from build123d import *

# Parameters (mm, degrees)
BOSS_EXTRUDE1_DEPTH     = 10
SKETCH4_W               = 12
SKETCH4_H               = 57
BOSS_EXTRUDE2_DEPTH     = 10
SKETCH3_R               = 1.3
CUT_EXTRUDE1_DEPTH      = 1
CUT_EXTRUDE1_DEPTH_BACK = 20.5


with BuildPart() as part:
    # Sketch2 → Boss-Extrude1 (new body)
    with BuildSketch(Plane(origin=(0, 0, 0), x_dir=(0, 0, -1), z_dir=(1, 0, 0))):
        with BuildLine():
            Line((27, 28.5), (7.5, 28.5))
            Line((7.5, 28.5), (7.5, 17.589059099))
            ThreePointArc((7.5, 17.589059099), (15, 0), (7.5, -17.589059099))
            Line((7.5, -17.589059099), (7.5, -28.5))
            Line((7.5, -28.5), (27, -28.5))
            Line((27, -28.5), (27, 28.5))
        make_face()
    boss_extrude1 = extrude(amount=BOSS_EXTRUDE1_DEPTH)

    # Sketch4 → Boss-Extrude2 (add)
    with BuildSketch(Plane.ZY):
        with Locations((-21, 0)):
            Rectangle(SKETCH4_W, SKETCH4_H)
    extrude(amount=BOSS_EXTRUDE2_DEPTH)

    # Mirror1: Boss-Extrude1 across plane
    add(boss_extrude1.mirror(Plane.ZY.offset(5)))

    # Sketch3 → Cut-Extrude1 (cut, two sides)
    with BuildSketch(Plane(origin=(0, 0, -27), x_dir=(-1, 0, 0), z_dir=(0, 0, -1))) as cut_extrude1_sk:
        with Locations((5, -22.5)):
            Circle(SKETCH3_R)
        with Locations((5, 22.5)):
            Circle(SKETCH3_R)
        with Locations((5, 0)):
            Circle(SKETCH3_R)
    extrude(amount=CUT_EXTRUDE1_DEPTH, mode=Mode.SUBTRACT)
    extrude(cut_extrude1_sk.sketch, amount=-CUT_EXTRUDE1_DEPTH_BACK, mode=Mode.SUBTRACT)


solid = part.part
The listing builds one solid part. Answer for the finished solid, in the listing's coordinates (mm). A direction names the side the tool comes from. Coordinates: 2 decimals unless noted, no trailing zeros. Loops run counter-clockwise (first coordinate to the right, second up) from the corner with the lowest first, then second, coordinate; pieces in that order, holes last. Notation, with made-up numbers: (48.5, 89.5) -> (77.5, 89.5) arc R22 ccw to (77.5, 106.5) -> close; hole circle Ø7 at (-1.5, 23). An arc over 180 degrees is marked (long way). Answer in a Markdown table with one row per item. Add a question column.
1. The part is cut by section A-A, the plane y = -22.5. Write down the section's boundary in (x, z), then the cut area to 3 significant figures.
2. For faces 4 (the flat face through (-10, 21, -12)), 5 (the cylindrical face through (-15, 0, -15)), determine the directions among +Z, -Z, +X, -X, +Y, -Y from which every point of the face is accessible in a straight line to the end or side of a thin tool.
3. The part is cut by section B-B, the plane y = -6. Write down the section's boundary in (x, z), then the cut area to 3 significant figures.
4. Determine the mould class of faces 1 (the flat face through (-15, -23, -7.5)), 2 (the flat face through (-5, 28.5, -17)), 3 (the cylindrical face through (-4.72, -23.77, -21.08)) for opening direction Y: +Y half, -Y half, draft (parallel to the pull), parting line (faces both ways), or undercut.
5. The part is cut by section D-D, the plane x = 1. Write down the section's boundary in (y, z) (3 decimals), then the cut area to 3 significant figures.
6. Consider line 1 (Y direction, x = -5, z = -23.5); line 2 (Y direction, x = -4, z = -25); line 3 (X direction, y = -22.5, z = -14.75). Determine where each line is inside the solid, lowest interval first. Write a range as [from, to].
7. Flat-ended cylindrical pins translate along their axes: P1, Ø5, axis at x = -4, y = 13, coming from the +Z side; P2, Ø2.5, axis at x = -5, y = 0, coming from the -Z side; P3, Ø12, axis at x = 0.5, y = 2, coming from the +Z side. Find the tip coordinate at first contact, or state that the pin passes through.
8. The part is cut by section C-C, the plane z = -10. Write down the section's boundary in (x, y).
Answer below:
| question | item | result |
|---|---|---|
| 1 | outline | (-20, -27) -> (-6.3, -27) -> (-6.3, -15) -> (-10, -15) -> (-10, -7.5) -> (-20, -7.5) -> close; (-3.7, -27) -> (10, -27) -> (10, -7.5) -> (0, -7.5) -> (0, -15) -> (-3.7, -15) -> close |
| 1 | area | 479 mm2 |
| 2 | face 4 | +Z, +Y, -Y |
| 2 | face 5 | +Z, +X, -X |
| 3 | outline | (-20, -27) -> (10, -27) -> (10, -14.25) -> (0, -14.25) -> (0, -15) -> (-10, -15) -> (-10, -14.25) -> (-20, -14.25) -> close |
| 3 | area | 375 mm2 |
| 4 | face 1 | draft |
| 4 | face 2 | +Y half |
| 4 | face 3 | undercut |
| 5 | outline | (-28.5, -27) -> (28.5, -27) -> (28.5, -7.5) -> (17.589, -7.5) arc R24.375 cw to (-17.589, -7.5) -> (-28.5, -7.5) -> close |
| 5 | area | 929 mm2 |
| 6 | line 1 | [-28.5, -23.8], [-21.2, -1.3], [1.3, 21.2], [23.8, 28.5] |
| 6 | line 2 | [-28.5, -23.33], [-21.67, -0.83], [0.83, 21.67], [23.33, 28.5] |
| 6 | line 3 | [-20, -10], [0, 10] |
| 7 | P1 | z = -15 |
| 7 | P2 | through |
| 7 | P3 | z = -13.65 |
| 8 | outline | (-20, -28.5) -> (-10, -28.5) -> (-10, -14.79) -> (-20, -14.79) -> close; (-20, 14.79) -> (-10, 14.79) -> (-10, 28.5) -> (-20, 28.5) -> close; (0, -28.5) -> (10, -28.5) -> (10, -14.79) -> (0, -14.79) -> close; (0, 14.79) -> (10, 14.79) -> (10, 28.5) -> (0, 28.5) -> close |
